```python
from build123d import *

# Parameters (mm, degrees)
SKETCH1_R           = 1.65
SKETCH1_W           = 19
SKETCH1_H           = 46
BOSS_EXTRUDE3_DEPTH = 5
SKETCH5_R           = 2.55
CUT_EXTRUDE2_DEPTH  = 90.162772501
SKETCH9_W           = 10.2
SKETCH9_H           = 15.2
CUT_EXTRUDE3_DEPTH  = 90.162772501
SKETCH6_W           = 30
SKETCH6_H           = 6
BOSS_EXTRUDE4_DEPTH = 50
SKETCH11_W          = 16
SKETCH11_H          = 10.2
CUT_EXTRUDE4_DEPTH  = 103.102889283


with BuildPart() as part:
    # Sketch1 → Boss-Extrude3 (new body)
    with BuildSketch(Plane(origin=(0, 0, 0), x_dir=(1, 0, 0), z_dir=(0, 1, 0))):
        Polygon((55, 50), (-55, 50), (-55, 31.75), (-55, -31.75), (-55, -70), (-20, -70), (2.5, -70), (20, -70), (42.5, -70), (55, -70), (55, -31.75), (55, 31.75), align=None)
        with Locations(Location((-29.5, -32, 0), (0, 0, 270))):
            Circle(SKETCH1_R, mode=Mode.SUBTRACT)
        with Locations(Location((-19.5, -32, 0), (0, 0, 270))):
            Circle(SKETCH1_R, mode=Mode.SUBTRACT)
        with Locations(Location((19.5, -32, 0), (0, 0, 270))):
            Circle(SKETCH1_R, mode=Mode.SUBTRACT)
        with Locations(Location((29.5, -32, 0), (0, 0, 270))):
            Circle(SKETCH1_R, mode=Mode.SUBTRACT)
        with Locations(Location((-29.5, 32, 0), (0, 0, 270))):
            Circle(SKETCH1_R, mode=Mode.SUBTRACT)
        with Locations(Location((-19.5, 32, 0), (0, 0, 270))):
            Circle(SKETCH1_R, mode=Mode.SUBTRACT)
        Rectangle(SKETCH1_W, SKETCH1_H, mode=Mode.SUBTRACT)
        with Locations(Location((19.5, 32, 0), (0, 0, 270))):
            Circle(SKETCH1_R, mode=Mode.SUBTRACT)
        with Locations(Location((29.5, 32, 0), (0, 0, 270))):
            Circle(SKETCH1_R, mode=Mode.SUBTRACT)
    extrude(amount=BOSS_EXTRUDE3_DEPTH)

    # Sketch5 → Cut-Extrude2 (cut, through all)
    with BuildSketch(Plane.XZ):
        with Locations(Location((-45, 60, 0), (0, 0, 270))):
            Circle(SKETCH5_R)
        with Locations(Location((-45, -35, 0), (0, 0, 270))):
            Circle(SKETCH5_R)
        with Locations(Location((45, -35, 0), (0, 0, 90))):
            Circle(SKETCH5_R)
        with Locations(Location((45, 60, 0), (0, 0, 90))):
            Circle(SKETCH5_R)
    extrude(amount=-CUT_EXTRUDE2_DEPTH, mode=Mode.SUBTRACT)

    # Sketch9 → Cut-Extrude3 (cut, through all)
    with BuildSketch(Plane(origin=(0, 5, 0), x_dir=(1, 0, 0), z_dir=(0, 1, 0))):
        with Locations((-19.6, 15.6)):
            Rectangle(SKETCH9_W, SKETCH9_H)
        with Locations((-19.6, -15.6)):
            Rectangle(SKETCH9_W, SKETCH9_H)
        with Locations((19.6, -15.6)):
            Rectangle(SKETCH9_W, SKETCH9_H)
        with Locations((19.6, 15.6)):
            Rectangle(SKETCH9_W, SKETCH9_H)
    extrude(amount=-CUT_EXTRUDE3_DEPTH, mode=Mode.SUBTRACT)

    # Sketch6 → Boss-Extrude4 (add)
    with BuildSketch(Plane(origin=(0, 5, 0), x_dir=(1, 0, 0), z_dir=(0, 1, 0))):
        with Locations((-20, -39)):
            Rectangle(SKETCH6_W, SKETCH6_H)
        with Locations((20, -39)):
            Rectangle(SKETCH6_W, SKETCH6_H)
    extrude(amount=BOSS_EXTRUDE4_DEPTH)

    # Sketch11 → Cut-Extrude4 (cut, through all)
    with BuildSketch(Plane(origin=(0, 5, 0), x_dir=(1, 0, 0), z_dir=(0, 1, 0))):
        with Locations((22.5, 0)):
            Rectangle(SKETCH11_W, SKETCH11_H)
    extrude(amount=-CUT_EXTRUDE4_DEPTH, mode=Mode.SUBTRACT)


solid = part.part
```
Could you check a few things on this model? Use its own coordinates, in mm. A direction names the side the tool comes from. Round coordinates to 2 decimals unless told otherwise and drop trailing zeros. Loops run counter-clockwise (first coordinate to the right, second up) from the corner with the lowest first, then second, coordinate; pieces in that order, holes last.
Q1. I want a section at D-D (y = 14.5). Write out the boundary of the cut face in (x, z).
Q2. On a 3-axis mill with a long thin cutter (end or side, diameter ignored), from which of +Z, -Z, +X, -X, +Y, -Y can I reach the whole of each face in a straight line? I mean faces 1 (the flat face through (-5, 30, 39)), 2 (the flat face through (55, 2, 11)), 3 (the flat face through (-20, 30, 36)), 4 (the flat face through (-20, 30, 42)), 5 (the flat face through (22, 3, -5.1)). Say none if no direction works.
Q3. I want a section at C-C (x = 19.5). Write out the boundary of the cut face in (y, z), and give its area (3 significant figures).
Q4. I want a section at A-A (x = -0.5). Write out the boundary of the cut face in (y, z).
Q5. Please list where these lines run through material, in increasing order: L1, parallel to X at y = 3.35, z = -32; L2, parallel to X at y = 3.6, z = -35; L3, parallel to Z at x = 45, y = 1.
Q6. For P1, Ø2, axis at x = -25, z = 5.5, coming from the -Y side; P2, Ø24, axis at x = 23, y = 38, coming from the -Z side; P3, Ø1.5, axis at y = 37, z = 35.5, coming from the +X side; P4, Ø6, axis at x = -8, z = -8, coming from the +Y side, each with a flat end and sliding along its axis, tell me the tip position at first contact or that it passes through.
Q7. I want a section at B-B (z = 60). Write out the boundary of the cut face in (x, y), and give its area (3 significant figures).
Answer below:
1. outline: (-35, 36) - (-5, 36) - (-5, 42) - (-35, 42) - close; (5, 36) - (35, 36) - (35, 42) - (5, 42) - close
2. face 1: +Z, -Z, +Y
2. face 2: +Z, -Z, +X, +Y, -Y
2. face 3: -Z, +X, -X, +Y
2. face 4: +Z, +X, -X, +Y
2. face 5: +Y, -Y
3. outline: (0, -50) - (5, -50) - (5, -33.65) - (0, -33.65) - close; (0, -30.35) - (5, -30.35) - (5, -23.2) - (0, -23.2) - close; (0, -8) - (5, -8) - (5, -5.1) - (0, -5.1) - close; (0, 5.1) - (5, 5.1) - (5, 8) - (0, 8) - close; (0, 23.2) - (5, 23.2) - (5, 30.35) - (0, 30.35) - close; (0, 33.65) - (5, 33.65) - (5, 36) - (55, 36) - (55, 42) - (5, 42) - (5, 70) - (0, 70) - close
3. area: 664 mm2
4. outline: (0, -50) - (5, -50) - (5, -23) - (0, -23) - close; (0, 23) - (5, 23) - (5, 70) - (0, 70) - close
5. L1: x = -55 to -31.15, -27.85 to -21.15, -17.85 to 17.85, 21.15 to 27.85, 31.15 to 55
5. L2: x = -55 to -47.55, -42.45 to 42.45, 47.55 to 55
5. L3: z = -50 to -37.55, -32.45 to 57.45, 62.55 to 70
6. P1: stops at y = 0
6. P2: stops at z = 36
6. P3: stops at x = 35
6. P4: stops at y = 5
7. outline: (-55, 0) - (-47.55, 0) - (-47.55, 5) - (-55, 5) - close; (-42.45, 0) - (42.45, 0) - (42.45, 5) - (-42.45, 5) - close; (47.55, 0) - (55, 0) - (55, 5) - (47.55, 5) - close
7. area: 499 mm2
